```python
from build123d import *

# Parameters (mm, degrees)
F0_R     = 41.275
F1_DEPTH = 89.916
F2_R     = 30.988
F3_DEPTH = 80.264
F5_DEPTH = 19.05


with BuildPart() as f1:
    # F0 (on Top) → F1 (new body)
    with BuildSketch(Plane.XY):
        Circle(F0_R)
    extrude(amount=F1_DEPTH)

    # F2 (on face) → F3 (cut)
    with BuildSketch(Plane.XY.offset(89.916)):
        Circle(F2_R)
    extrude(amount=-F3_DEPTH, mode=Mode.SUBTRACT)

    # F4 (on face) → F5 (cut)
    with BuildSketch(Plane.XY.offset(89.916)):
        Polygon((3.175, 33.36925), (0, 33.36925), (-3.175, 33.36925), (-3.175, 0), (-3.175, -33.36925), (0, -33.36925), (3.175, -33.36925), (3.175, 0), align=None)
    extrude(amount=-F5_DEPTH, mode=Mode.SUBTRACT)


solid = f1.part
```
Here's how the part is built. I have some questions about the finished solid (model axes, mm). A direction names the side the tool comes from. Round coordinates to 2 decimals unless told otherwise and drop trailing zeros. Order: outer loops, then holes, each group sorted by start corner. A loop starts at its lowest first (then second) coordinate and runs counter-clockwise, first axis right, second up. Notation, with made-up numbers: (70, 27.5) -> (103, 27.5) arc R27 ccw to (103, 58.5) -> close; hole circle Ø10 at (37.5, 35). An arc over 180 degrees is marked (long way). Use a Markdown table: item, result. Add a question column.
(1) Suppose I cut it at C-C, the plane x = 0. Please give me the cut outline in (y, z) (3 decimals), and give its area (3 significant figures).
(2) If we mould it in two halves opening along X, with no side actions, what happens to faces 3 (the face through (0, 0, 9.652)), 4 (the face through (-1, 1, 0)), 5 (the face through (3.175, -32, 81)), 6 (the face through (-8.948, -40.293, 44.329))? For each: released by +X, released by -X, zero draft, split by the parting line, or undercut.
(3) Suppose I cut it at A-A, the plane z = 73. Please give me the cut outline in (x, y) (3 decimals).
(4) I need wall thicknesses on line 1 along Y through (x, z) = (0, 47) (3 decimals); line 2 along Z through (x, y) = (-16, 3); line 3 along Y through (x, z) = (-21, 25.5). Which ranges of each line are inside material? Lowest first, please.
(5) Suppose I cut it at B-B, the plane y = 0. Please give me the cut outline in (x, z) (3 decimals), and give its area (3 significant figures).
(6) For faces 1 (the face through (0, -33.369, 81)), 2 (the face through (6, 31, 89.916)), which set-ups out of +Z, -Z, +X, -X, +Y, -Y let a thin tool reach every point of the face, with its end or its side?
(7) Suppose I cut it at D-D, the plane y = 27. Please give me the cut outline in (x, z).
(8) For pin 1 Ø2 at (x, y) = (-0.5, -31.5) entering from +Z; pin 2 Ø18.5 at (x, y) = (12.5, 14) entering from +Z; pin 3 Ø1.3 at (y, z) = (32.5, 80.5) entering from +X, each with a flat end and sliding along its axis, tell me the tip position at first contact or that it passes through.
Verdict:
| question | item | result |
|---|---|---|
| 1 | outline | (-41.275, 0) -> (41.275, 0) -> (41.275, 89.916) -> (33.369, 89.916) -> (33.369, 70.866) -> (30.988, 70.866) -> (30.988, 9.652) -> (-30.988, 9.652) -> (-30.988, 70.866) -> (-33.369, 70.866) -> (-33.369, 89.916) -> (-41.275, 89.916) -> close |
| 1 | area | 2,360 mm2 |
| 2 | face 3 | undercut |
| 2 | face 4 | zero draft |
| 2 | face 5 | undercut |
| 2 | face 6 | split by the parting line |
| 3 | outline | circle Ø82.55 at (0, 0); hole (-3.175, -33.369) -> (3.175, -33.369) -> (3.175, -30.825) arc R30.988 ccw to (3.175, 30.825) -> (3.175, 33.369) -> (-3.175, 33.369) -> (-3.175, 30.825) arc R30.988 ccw to (-3.175, -30.825) -> close |
| 4 | line 1 | -41.275 to -30.988, 30.988 to 41.275 |
| 4 | line 2 | 0 to 9.65 |
| 4 | line 3 | -35.53 to -22.79, 22.79 to 35.53 |
| 5 | outline | (-41.275, 0) -> (41.275, 0) -> (41.275, 89.916) -> (30.988, 89.916) -> (30.988, 9.652) -> (-30.988, 9.652) -> (-30.988, 89.916) -> (-41.275, 89.916) -> close |
| 5 | area | 2,450 mm2 |
| 6 | face 1 | +Z |
| 6 | face 2 | +Z, +X, -X, +Y, -Y |
| 7 | outline | (-31.22, 0) -> (31.22, 0) -> (31.22, 89.92) -> (15.21, 89.92) -> (15.21, 9.65) -> (-15.21, 9.65) -> (-15.21, 89.92) -> (-31.22, 89.92) -> close |
| 8 | pin 1 | z = 70.87 |
| 8 | pin 2 | z = 9.65 |
| 8 | pin 3 | x = 26.25 |
